Verification items for the finished model (mm, model axes). A direction names the side the tool comes from. Coordinates: 2 decimals unless noted, no trailing zeros. Loops run counter-clockwise (first coordinate to the right, second up) from the corner with the lowest first, then second, coordinate; pieces in that order, holes last. Notation, with made-up numbers: (14, 24.5) - (41, 24.5) arc R18 cw to (41, 33.5) - close; hole circle Ø7 at (46.25, -39.75). An arc over 180 degrees is marked (long way). Answer as CSV lines item,"result". Start each with the question number.
1. Set-up check for faces 4 (the flat face through (-3, 9, 6)), 5 (the flat face through (0, 17, 1.702)), 6 (the flat face through (1.588, 1, 0)): record each of +Z, -Z, +X, -X, +Y, -Y from which the full face is reachable in a straight line by a thin tool's end or side.
2. Release check for a two-part mould opening along Z. For faces 1 (the cylindrical face through (-10.54, 17.19, 11.76)), 2 (the flat face through (5, 8, 7)), 3 (the flat face through (0, 17, 26.702)) record: pulls with the +Z half, pulls with the -Z half, needs draft (parallel to the pull), parting line crosses it, or undercut.
3. Cross-section at A-A (z = 0.5). Enter the section's corners in (x, y), plus the area to 4 significant figures.
4. Material ranges on line 1 (X direction, y = 10.25, z = 7); line 2 (X direction, y = 1.25, z = 4); line 3 (Y direction, x = 10, z = 19.5), recorded low to high. Write a range as [from, to].
5. Cross-section at D-D (z = 11). Enter the section's corners in (x, y).
6. Cross-section at C-C (y = 4.5). Enter the section's corners in (x, z), plus the area to 3 significant figures.
7. Gauge pin test, flat ends, axial feed: P1, Ø1, axis at x = 4.5, z = 15, coming from the -Y side; P2, Ø11, axis at x = 11, z = 16, coming from the -Y side; P3, Ø4, axis at y = 13.5, z = 2.5, coming from the +X side. Record the tip position at first contact, or that the pin passes through.
Autodesk Inventor part; units mm, degrees
ref_plane "YZ Plane" through (0, 0, 0) normal (1, 0, 0) x (0, 1, 0)
ref_plane "XZ Plane" through (0, 0, 0) normal (0, 1, 0) x (-1, 0, 0)
ref_plane "XY Plane" through (0, 0, 0) normal (0, 0, 1) x (1, 0, 0)
sketch "Sketch1" plane through (0, 0, 0) normal (0, 1, 0) x (-1, 0, 0)
  line L0 (5, 12.5) -> (-5, 12.5)
  line L1 (-5, 12.5) -> (-5, -12.5)
  line L2 (-5, -12.5) -> (5, -12.5)
  line L3 (5, -12.5) -> (5, 12.5)
  line L4 (5, 12.5) -> (-5, -12.5) construction
  line L5 (-5, 12.5) -> (5, -12.5) construction
  line L6 (0, 7.5) -> (0, -7.5) construction
  line L7 (-1.5875, 7.5) -> (-1.5875, -7.5)
  line L8 (1.5875, -7.5) -> (1.5875, 7.5)
  arc A0 (1.5875, 7.5) -> (-1.5875, 7.5) centre (0, 7.5) ccw
  arc A1 (-1.5875, -7.5) -> (1.5875, -7.5) centre (0, -7.5) ccw
  point P0 (0, 0)
  point P1 (0, 0)
  dimension "d0" = 10
  dimension "d1" = 25
  dimension "d2" = 7.5
  dimension "d3" = 7.5
  dimension "d4" = 3.175
extrude "Extrusion1" add sketch "Sketch1" along normal blind 2
sketch "Sketch2" plane through (0, 2, 0) normal (0, 1, 0) x (1, 0, 0)
  line L0 (5, -12.5) -> (5, 12.5)
  line L1 (5, 12.5) -> (-5, 12.5)
  line L2 (-5, 12.5) -> (-5, -12.5)
  line L3 (-5, -12.5) -> (5, -12.5)
  arc A0 (-1.5875, -7.5) -> (1.5875, -7.5) centre (0, -7.5) ccw
  line L4 (-1.5875, -7.5) -> (-1.5875, 7.5)
  arc A1 (1.5875, 7.5) -> (-1.5875, 7.5) centre (0, 7.5) ccw
  line L5 (1.5875, 7.5) -> (1.5875, -7.5)
  line L6 (-3, -10.5) -> (-3, 10.5)
  line L7 (3, 10.5) -> (3, -10.5)
  line L8 (3, -10.5) -> (-3, -10.5)
  line L9 (-3, 10.5) -> (-3, 12.5)
  line L10 (3, 10.5) -> (3, 12.5)
  point P0 (0, 0)
  dimension "d7" = 2
sketch "Sketch3" plane through (0, 0, 0) normal (1, 0, 0) x (0, 1, 0)
  line L0 (2, 12.5) -> (16.2024, 26.7024)
  point P0 (0, 0)
  dimension "d15" = 20.0852
sweep "Sweep1" add profiles "Sketch2" path "Sketch3" contours L3 L2 L1 L9 L6 L8 L7 L10 L0
chamfer "Chamfer1" distance 2 angle 45 1 edges at (0, 0, 12.5)
sketch "Sketch5" plane through (-5, 16.2024, 26.7024) normal (0, 1, 0) x (1, 0, 0)
  line L0 (20, 0) -> (-10, 0)
  line L1 (-10, 0) -> (-10, 25)
  line L2 (-10, 25) -> (20, 25)
  line L3 (20, 25) -> (20, 0)
  line L4 (10, 0) -> (10, 25)
  circle A0 centre (15, 12.5) radius 2.5
  circle A1 centre (-5, 12.5) radius 2.5
  point P0 (5, 26.7024)
  dimension "d23" = 25
  dimension "d24" = 30
  dimension "d25" = 10
  dimension "d26" = 5
  dimension "d27" = 5
  dimension "d28" = 5
  dimension "d29" = 5
extrude "Extrusion4" add sketch "Sketch5" along normal blind 2
fillet "Fillet1" radius 10 4 edges at (15, 17.2024, 1.7024) (-15, 17.2024, 1.7024) (-15, 17.2024, 26.7024) (15, 17.2024, 26.7024)
properties part number "ancla"
Values follow:
1,face 4,"-Z"
1,face 5,"-Z, +X, -X, +Y"
1,face 6,"-Y"
2,face 1,"undercut"
2,face 2,"needs draft"
2,face 3,"pulls with the +Z half"
3,outline,"(-5, 0) - (-1.59, 0) - (-1.59, 2) - (-3, 2) - (-3, 15) - (-5, 15) - close; (1.59, 0) - (5, 0) - (5, 15) - (3, 15) - (3, 2) - (1.59, 2) - close"
3,area,"65.65 mm²"
4,line 1,"x = [-5, -3], [3, 5]"
4,line 2,"x = [-5, -1.59], [1.59, 5]"
4,line 3,"y = [16.2, 18.2]"
5,outline,"(-14.98, 16.2) - (-5, 16.2) - (-5, 0.5) - (5, 0.5) - (5, 16.2) - (14.98, 16.2) - (14.98, 18.2) - (-14.98, 18.2) - close; hole (-3, 2.5) - (3, 2.5) - (3, 16.2) - (-3, 16.2) - close"
6,outline,"(-5, -10) - (-3, -10) - (-3, 13) - (3, 13) - (3, -10) - (5, -10) - (5, 15) - (-5, 15) - close"
6,area,"112 mm²"
7,P1,"stops at y = 4"
7,P2,"stops at y = 16.2"
7,P3,"stops at x = 5"
